Verification items for the finished model (mm, model axes). Round coordinates to 2 decimals unless told otherwise and drop trailing zeros. Order: outer loops, then holes, each group sorted by start corner. A loop starts at its lowest first (then second) coordinate and runs counter-clockwise, first axis right, second up. Notation, with made-up numbers: (23.25, 27.25) -> (40.25, 27.25) arc R25 ccw to (40.25, 61.25) -> close; hole circle Ø1 at (-36.5, 18.5). An arc over 180 degrees is marked (long way). Return JSON: item names as keys, results as strings. Group by question number.
1) Scan lines: L1, parallel to X at y = 0.65, z = 8.5; L2, parallel to Z at x = 4.75, y = 2.4; L3, parallel to Z at x = 5, y = 1.6. Record each from-to range of solid material in increasing order.
2) Section check D-D on y = 0.9. State how many separate pieces and enclosed holes the cut face has, plus the area to 3 significant figures.
3) Section check A-A on z = 0. Enter the section's corners in (x, y) (3 decimals).
4) Section check C-C on z = -6.5. Enter the section's corners in (x, y).
5) Draft check along Z on faces 1 (the cylindrical face through (-7.62, 1.23, 3.16)), 2 (the cylindrical face through (-5.697, 1.232, 8.282)), 3 (the flat face through (7, 1.5, 10)), 4 (the cylindrical face through (11.99, 1.99, -0.53)). Enter one of: pulls with the +Z half, pulls with the -Z half, needs draft (parallel to the pull), parting line crosses it, or undercut.
6) Section check B-B on x = 0. Enter the section's corners in (y, z), plus the area to 4 significant figures.
7) Depth check by flat-ended pin: pin 1 (2.5 mm diameter, centred on x = -5.06, z = -8.77, fed in from -Y); pin 2 (1 mm diameter, centred on x = -3, y = 1, fed in from -Z); pin 3 (1.5 mm diameter, centred on x = -9.5, y = 0.5, fed in from -Z); pin 4 (1 mm diameter, centred on x = 9.5, y = 1, fed in from -Z). Enter the tip coordinate at first touch or a pass-through.
Autodesk Inventor part; units mm, degrees
ref_plane "YZ Plane" through (0, 0, 0) normal (1, 0, 0) x (0, 1, 0)
ref_plane "XZ Plane" through (0, 0, 0) normal (0, 1, 0) x (-1, 0, 0)
ref_plane "XY Plane" through (0, 0, 0) normal (0, 0, 1) x (1, 0, 0)
sketch "スケッチ1" plane through (0, 0, 0) normal (0, 1, 0) x (-1, 0, 0)
  circle A0 centre (0, 0) radius 8.25
  circle A1 centre (0, 0) radius 15
  circle A2 centre (0, 0) radius 12
  dimension "d0" = 16.5
  dimension "d1" = 30
  dimension "d5" = 24
extrude "押し出し1" add sketch "スケッチ1" along normal blind 1.5 contours A1 | A2
extrude "押し出し2" add sketch "スケッチ1" along normal blind 2.5 contours A2
sketch "スケッチ2" plane through (0, 0, 0) normal (0, -1, 0) x (1, 0, 0)
  circle A0 centre (5.0625, -8.7685) radius 1 construction
  circle A1 centre (10.125, 0) radius 1 construction
  circle A2 centre (5.0625, 8.7685) radius 1 construction
  circle A3 centre (-5.0625, 8.7685) radius 1 construction
  circle A4 centre (-10.125, 0) radius 1 construction
  circle A5 centre (-5.0625, -8.7685) radius 1 construction
  circle A6 centre (10.125, 0) radius 0.8
  circle A7 centre (5.0625, -8.7685) radius 0.8
  circle A8 centre (-5.0625, -8.7685) radius 0.8
  circle A9 centre (-10.125, 0) radius 0.8
  circle A10 centre (-5.0625, 8.7685) radius 0.8
  circle A11 centre (5.0625, 8.7685) radius 0.8
  point P0 (0, 0)
  dimension "d10" = 1.6
  dimension "d11" = 1.6
  dimension "d12" = 1.6
  dimension "d13" = 1.6
  dimension "d14" = 1.6
  dimension "d15" = 1.6
extrude "押し出し3" cut sketch "スケッチ2" against normal through all
equation "\"BendRadius\" = Thickness"
equation "\"BendReliefWidth\" = Thickness"
equation "\"BendReliefDepth\" = 0.5 * Thickness"
equation "\"CornerReliefSize\" = 4 * Thickness"
equation "\"MinimumRemnant\" = 2 * Thickness"
equation "\"TransitionRadius\" = BendRadius"
equation "\"JacobiRadiusSize\" = BendRadius"
equation "\"GapSize\" = Thickness"
properties part number "sholder_joint_c"
Check result:
{
 "1": {"L1": "-12.36 to -5.82, -4.31 to 4.31, 5.82 to 12.36", "L2": "-11.02 to -9.5, -8.03 to -6.75, 6.75 to 8.03, 9.5 to 11.02", "L3": "-10.91 to -9.57, -7.97 to -6.56, 6.56 to 7.97, 9.57 to 10.91"},
 "2": {"separate pieces": "1", "enclosed holes": "7", "area": "481 mm^2"},
 "3": {"outline": "(-15, 0) -> (-10.925, 0) -> (-10.925, 2.5) -> (-12, 2.5) -> (-12, 1.5) -> (-15, 1.5) -> close; (-9.325, 0) -> (-8.25, 0) -> (-8.25, 2.5) -> (-9.325, 2.5) -> close; (8.25, 0) -> (9.325, 0) -> (9.325, 2.5) -> (8.25, 2.5) -> close; (10.925, 0) -> (15, 0) -> (15, 1.5) -> (12, 1.5) -> (12, 2.5) -> (10.925, 2.5) -> close"},
 "4": {"outline": "(-13.52, 0) -> (-5.08, 0) -> (-5.08, 2.5) -> (-10.09, 2.5) -> (-10.09, 1.5) -> (-13.52, 1.5) -> close; (5.08, 0) -> (13.52, 0) -> (13.52, 1.5) -> (10.09, 1.5) -> (10.09, 2.5) -> (5.08, 2.5) -> close"},
 "5": {"face 1": "undercut", "face 2": "undercut", "face 3": "needs draft", "face 4": "parting line crosses it"},
 "6": {"outline": "(0, -15) -> (1.5, -15) -> (1.5, -12) -> (2.5, -12) -> (2.5, -8.25) -> (0, -8.25) -> close; (0, 8.25) -> (2.5, 8.25) -> (2.5, 12) -> (1.5, 12) -> (1.5, 15) -> (0, 15) -> close", "area": "27.75 mm^2"},
 "7": {"pin 1": "y = 0", "pin 2": "z = -14.79", "pin 3": "z = -12.18", "pin 4": "z = -12"}
}
